from build123d import *

# Parameters (mm, degrees)
SKETCH2_R           = 10
BOSS_EXTRUDE2_DEPTH = 15


with BuildPart() as part:
    # Sketch2 → Boss-Extrude2 (new body)
    with BuildSketch(Plane.XY):
        with BuildLine():
            Line((-230, 27), (230, 27))
            ThreePointArc((230, 27), (257, 0), (230, -27))
            Line((230, -27), (-230, -27))
            Line((-230, -27), (-230, 27))
        make_face()
        with Locations(Location((230, 0, 0), (0, 0, 180))):
            Circle(SKETCH2_R, mode=Mode.SUBTRACT)
        with Locations((-205, 0)):
            Circle(SKETCH2_R, mode=Mode.SUBTRACT)
    extrude(amount=-BOSS_EXTRUDE2_DEPTH)


solid = part.part
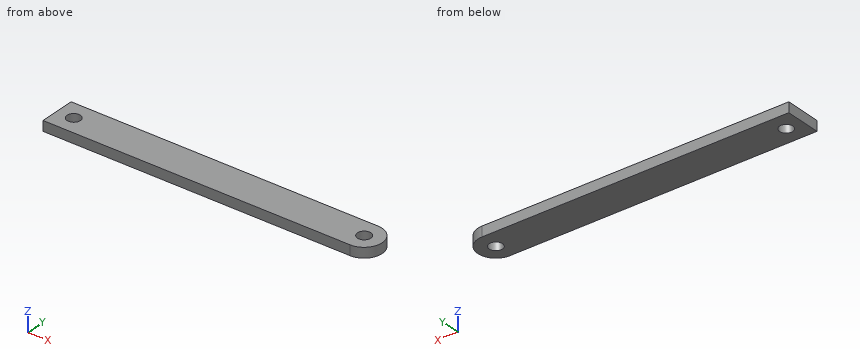
Source: CAD feature listing. Evaluate the final solid. Frame: model axes, mm. Round coordinates to 2 decimals unless told otherwise and drop trailing zeros. Write each loop counter-clockwise with the first axis right and the second up, starting at its lowest first coordinate (ties: lowest second). Pieces come first, ordered by that corner, then holes. Notation, with made-up numbers: M -33.5,74 L 1.5,74 A21 cw 1.5,95 Z; hole C 80,-34.5 d7. An arc over 180 degrees is marked long. One line per item, written item: value. Start each with the question number.
Item 1: Section query C-C (z = -4). Return the cut outline in (x, y).
Item 2: Section query A-A (y = 0). Return the cut outline in (x, z), plus the area to 4 significant figures.
Item 3: Pin query (flat end, axial travel): pin 1 (3 mm diameter, centred on y = 3.5, z = -6.5, fed in from +X); pin 2 (5 mm diameter, centred on y = 10.5, z = -4.5, fed in from +X). Return the tip coordinate at first contact, or that it passes through.
Item 4: Ray query, L1, parallel to X at y = 1, z = -1.75; L2, parallel to Y at x = 230, z = -8.25; L3, parallel to X at y = 3.5, z = -5. Return the intervals inside material, ascending. Write a range as from..to.
Item 5: Section query B-B (x = -205). Return the cut outline in (y, z).
Result set:
1. outline: M -230,-27 L 230,-27 A27 ccw 230,27 L -230,27 Z; hole C -205,0 d20; hole C 230,0 d20
2. outline: M -230,-15 L -215,-15 L -215,0 L -230,0 Z; M -195,-15 L 220,-15 L 220,0 L -195,0 Z; M 240,-15 L 257,-15 L 257,0 L 240,0 Z
2. area: 6,705 mm²
3. pin 1: stops at x = 256.93
3. pin 2: stops at x = 255.79
4. L1: x = -230..-214.95, -195.05..220.05, 239.95..256.98
4. L2: y = -27..-10, 10..27
4. L3: x = -230..-214.37, -195.63..220.63, 239.37..256.77
5. outline: M -27,-15 L -10,-15 L -10,0 L -27,0 Z; M 10,-15 L 27,-15 L 27,0 L 10,0 Z
